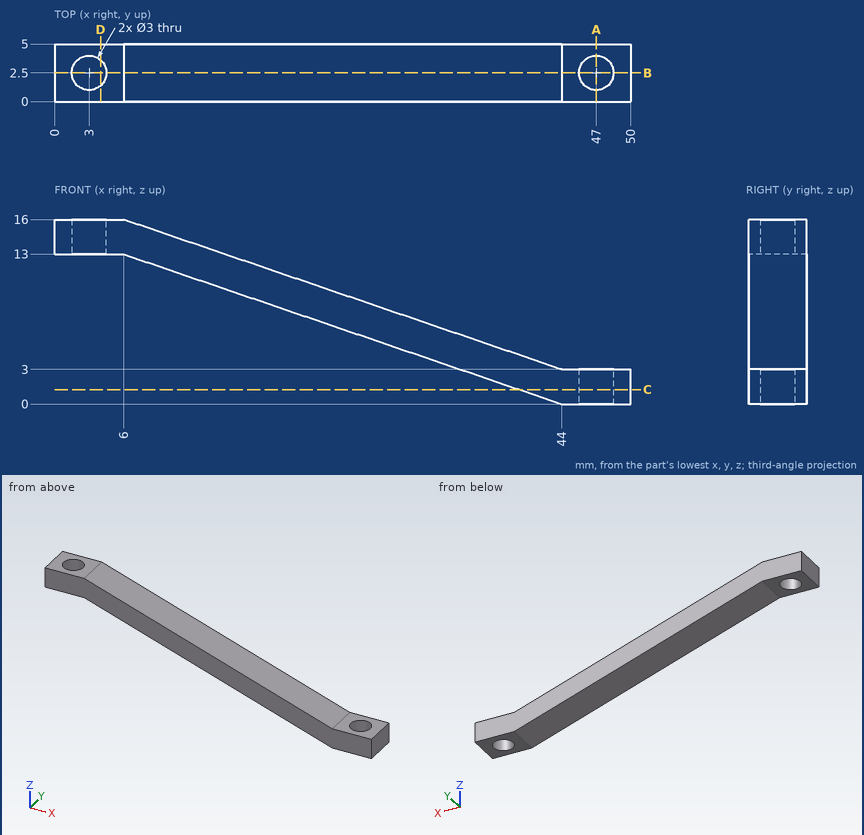
Input: dimensioned drawing with shaded views. Units: mm. Origin: part minimum x, y, z. Round coordinates to 2 decimals unless told otherwise and drop trailing zeros. Loops run counter-clockwise (first coordinate to the right, second up) from the corner with the lowest first, then second, coordinate; pieces in that order, holes last. Notation, with made-up numbers: M -11,26 L 2,26 A19 ccw 2,63 Z; hole C -14.75,31 d1. An arc over 180 degrees is marked long. One line per question, with ' | ' between items.
(1) Cut plane C-C on z = 1.25. Return the cut outline in (x, y), plus the area to 3 significant figures.
Check result:
outline: M 40.35,0 L 50,0 L 50,5 L 40.35,5 Z; hole C 47,2.5 d3 | area: 41.2 mm2
(2) Cut plane B-B on y = 2.5. Return the cut outline in (x, z).
Check result:
outline: M 0,13 L 1.5,13 L 1.5,16 L 0,16 Z; M 4.5,13 L 6,13 L 44,0 L 45.5,0 L 45.5,3 L 44,3 L 6,16 L 4.5,16 Z; M 48.5,0 L 50,0 L 50,3 L 48.5,3 Z
(3) Cut plane D-D on x = 4. Return the cut outline in (y, z), plus the area to 3 significant figures.
Check result:
outline: M 0,13 L 1.38,13 L 1.38,16 L 0,16 Z; M 3.62,13 L 5,13 L 5,16 L 3.62,16 Z | area: 8.29 mm2
(4) Contact query for flat-ended pins moving along their axis: P1, Ø2.5, axis at x = 3.5, y = 2, coming from the -Z side; P2, Ø2, axis at x = 24.5, y = 1.5, coming from the +Z side. Output: stop coordinate, or through.
Check result:
P1: stops at z = 13 | P2: stops at z = 10.01
(5) Cut plane A-A on x = 47. Return the cut outline in (y, z).
Check result:
outline: M 0,0 L 1,0 L 1,3 L 0,3 Z; M 4,0 L 5,0 L 5,3 L 4,3 Z
(6) Material intervals for line 1 along Y through (x, z) = (3, 13.8); line 2 along Z through (x, y) = (48.5, 4.25); line 3 along Z through (x, y) = (2.5, 4.35), sorted ascending. Write a range as from..to.
Check result:
line 1: y = 0..1, 4..5 | line 2: z = 0..3 | line 3: z = 13..16
